from build123d import *

# Parameters (mm, degrees)
SKETCH_1_W          = 800
SKETCH_1_H          = 80
SKETCH_1_R          = 3.3
SKETCH_1_R_2        = 2.75
SKETCH_1_R_3        = 10.5
EXTRUDE_1_DEPTH     = 5
SKETCH_2_W          = 50
SKETCH_2_H          = 80
CUT_EXTRUDE_1_DEPTH = 403.026118555


with BuildPart() as part:
    # 草图1 → 凸台-拉伸1 (new body)
    with BuildSketch(Plane.XY):
        Rectangle(SKETCH_1_W, SKETCH_1_H)
        with Locations((-318.384776311, 18.384776311)):
            Circle(SKETCH_1_R, mode=Mode.SUBTRACT)
        with Locations((-281.615223689, 18.384776311)):
            Circle(SKETCH_1_R, mode=Mode.SUBTRACT)
        with Locations((-281.615223689, -18.384776311)):
            Circle(SKETCH_1_R, mode=Mode.SUBTRACT)
        with Locations((-318.384776311, -18.384776311)):
            Circle(SKETCH_1_R, mode=Mode.SUBTRACT)
        with Locations((-215.202795796, 15.202795796)):
            Circle(SKETCH_1_R_2, mode=Mode.SUBTRACT)
        with Locations((-184.797204204, 15.202795796)):
            Circle(SKETCH_1_R_2, mode=Mode.SUBTRACT)
        with Locations((-184.797204204, -15.202795796)):
            Circle(SKETCH_1_R_2, mode=Mode.SUBTRACT)
        with Locations((-215.202795796, -15.202795796)):
            Circle(SKETCH_1_R_2, mode=Mode.SUBTRACT)
        with Locations((-200, 0)):
            Circle(SKETCH_1_R_3, mode=Mode.SUBTRACT)
        with Locations((-18.384776311, 18.384776311)):
            Circle(SKETCH_1_R, mode=Mode.SUBTRACT)
        with Locations((18.384776311, 18.384776311)):
            Circle(SKETCH_1_R, mode=Mode.SUBTRACT)
        with Locations((18.384776311, -18.384776311)):
            Circle(SKETCH_1_R, mode=Mode.SUBTRACT)
        with Locations((-18.384776311, -18.384776311)):
            Circle(SKETCH_1_R, mode=Mode.SUBTRACT)
        with Locations(Location((215.202795796, -15.202795796, 0), (0, 0, 180))):
            Circle(SKETCH_1_R_2, mode=Mode.SUBTRACT)
        with Locations(Location((184.797204204, -15.202795796, 0), (0, 0, 180))):
            Circle(SKETCH_1_R_2, mode=Mode.SUBTRACT)
        with Locations(Location((184.797204204, 15.202795796, 0), (0, 0, 180))):
            Circle(SKETCH_1_R_2, mode=Mode.SUBTRACT)
        with Locations(Location((215.202795796, 15.202795796, 0), (0, 0, 180))):
            Circle(SKETCH_1_R_2, mode=Mode.SUBTRACT)
        with Locations(Location((200, 0, 0), (0, 0, 180))):
            Circle(SKETCH_1_R_3, mode=Mode.SUBTRACT)
        with Locations(Location((318.384776311, -18.384776311, 0), (0, 0, 180))):
            Circle(SKETCH_1_R, mode=Mode.SUBTRACT)
        with Locations(Location((281.615223689, -18.384776311, 0), (0, 0, 180))):
            Circle(SKETCH_1_R, mode=Mode.SUBTRACT)
        with Locations(Location((281.615223689, 18.384776311, 0), (0, 0, 180))):
            Circle(SKETCH_1_R, mode=Mode.SUBTRACT)
        with Locations(Location((318.384776311, 18.384776311, 0), (0, 0, 180))):
            Circle(SKETCH_1_R, mode=Mode.SUBTRACT)
        with Locations((-100, 25)):
            Circle(SKETCH_1_R_2, mode=Mode.SUBTRACT)
        with Locations((-100, 0)):
            Circle(SKETCH_1_R_2, mode=Mode.SUBTRACT)
        with Locations((-100, -25)):
            Circle(SKETCH_1_R_2, mode=Mode.SUBTRACT)
        with Locations(Location((100, -25, 0), (0, 0, 180))):
            Circle(SKETCH_1_R_2, mode=Mode.SUBTRACT)
        with Locations(Location((100, 0, 0), (0, 0, 180))):
            Circle(SKETCH_1_R_2, mode=Mode.SUBTRACT)
        with Locations(Location((100, 25, 0), (0, 0, 180))):
            Circle(SKETCH_1_R_2, mode=Mode.SUBTRACT)
        with Locations((-300, 0)):
            Circle(SKETCH_1_R_3, mode=Mode.SUBTRACT)
        Circle(SKETCH_1_R_3, mode=Mode.SUBTRACT)
        with Locations(Location((300, 0, 0), (0, 0, 180))):
            Circle(SKETCH_1_R_3, mode=Mode.SUBTRACT)
    extrude(amount=EXTRUDE_1_DEPTH)

    # 草图2 → 切除-拉伸1 (cut, through all)
    with BuildSketch(Plane.XY.offset(5)):
        with Locations((-375, 0)):
            Rectangle(SKETCH_2_W, SKETCH_2_H)
        with Locations((375, 0)):
            Rectangle(SKETCH_2_W, SKETCH_2_H)
    extrude(amount=-CUT_EXTRUDE_1_DEPTH, mode=Mode.SUBTRACT)


solid = part.part
Verification items for the finished model (mm, model axes). Give positions to 0.01 mm unless a question says otherwise; leave off trailing zeros. Write each loop counter-clockwise with the first axis right and the second up, starting at its lowest first coordinate (ties: lowest second). Pieces come first, ordered by that corner, then holes.
(1) Material ranges on line 1 (Y direction, x = -184, z = 1.5); line 2 (Y direction, x = -100, z = 2.95); line 3 (Y direction, x = 202, z = 4.25), recorded low to high.
(2) Cross-section at C-C (z = 1.9). State how many separate pieces and enclosed holes the cut face has, plus the area to 3 significant figures.
(3) Cross-section at A-A (x = 200). Enter the section's corners in (y, z), plus the area to 3 significant figures.
(4) Gauge pin test, flat ends, axial feed: pin 1 (9 mm diameter, centred on x = 184.8, y = -15.2, fed in from -Z); pin 2 (3.5 mm diameter, centred on x = 215.2, y = -15.2, fed in from -Z). Record the tip position at first contact, or that the pin passes through.
(5) Cross-section at B-B (x = -297.5). Enter the section's corners in (y, z), plus the area to 3 significant figures.
(6) Mould release check, pull along X, two halves, no side actions. Record for faces 1 (the face through (10, 3.2, 2.5)), 2 (the face through (-5, 18, 5)): +X half, -X half, draft (parallel to the pull), parting line (faces both ways), or undercut.
Worked out:
1. line 1: y = -40 to -17.83, -12.57 to 12.57, 17.83 to 40
1. line 2: y = -40 to -27.75, -22.25 to -2.75, 2.75 to 22.25, 27.75 to 40
1. line 3: y = -40 to -10.31, 10.31 to 40
2. separate pieces: 1
2. enclosed holes: 31
2. area: 53,500 mm2
3. outline: (-40, 0) - (-10.5, 0) - (-10.5, 5) - (-40, 5) - close; (10.5, 0) - (40, 0) - (40, 5) - (10.5, 5) - close
3. area: 295 mm2
4. pin 1: stops at z = 0
4. pin 2: passes through
5. outline: (-40, 0) - (-10.2, 0) - (-10.2, 5) - (-40, 5) - close; (10.2, 0) - (40, 0) - (40, 5) - (10.2, 5) - close
5. area: 298 mm2
6. face 1: undercut
6. face 2: draft
